from build123d import *

# Parameters (mm, degrees)
F0_W     = 25
F0_H     = 25
F1_DEPTH = 25
F3_R     = 5
F4_R     = 5


with BuildPart() as f1:
    # F0 (on Top) → F1 (new body)
    with BuildSketch(Plane.XY):
        with Locations((89.836757, -287.5)):
            Rectangle(F0_W, F0_H)
        with Locations((89.836757, -237.5)):
            Rectangle(F0_W, F0_H)
        with Locations((89.836757, -187.5)):
            Rectangle(F0_W, F0_H)
        with Locations((89.836757, -137.5)):
            Rectangle(F0_W, F0_H)
        with Locations((89.836757, -87.5)):
            Rectangle(F0_W, F0_H)
        with Locations((89.836757, -37.5)):
            Rectangle(F0_W, F0_H)
        Polygon((77.336757, 0), (-297.663243, 0), (-297.663243, -25), (-285.163243, -25), (-285.163243, -60), (-297.663243, -60), (-297.663243, -265), (-285.163243, -265), (-285.163243, -300), (-297.663243, -300), (-297.663243, -325), (77.336757, -325), (77.336757, -300), (77.336757, -275), (77.336757, -250), (77.336757, -225), (77.336757, -200), (77.336757, -175), (77.336757, -150), (77.336757, -125), (77.336757, -100), (77.336757, -75), (77.336757, -50), (77.336757, -25), align=None)
    extrude(amount=F1_DEPTH)

    # F2: F1 across face


with BuildPart() as f1_1:
    add(f1.part)
    add(f1.part.mirror(Plane(origin=(-297.663243, -162.5, 12.5), x_dir=(0, -1, 0), z_dir=(-1, 0, 0))))

    # F3
    f3_edges = [f1_1.edges().sort_by_distance(p)[0] for p in [
        (-297.663243, 0, 25),
    ]]
    fillet(f3_edges, radius=F3_R)

    # F4
    f4_edges = [f1_1.edges().sort_by_distance(p)[0] for p in [
        (-297.663243, -325, 25),
    ]]
    fillet(f4_edges, radius=F4_R)


solid = f1_1.part
Source: CAD feature listing. Evaluate the final solid. Frame: model axes, mm. A direction names the side the tool comes from. Round coordinates to 2 decimals unless told otherwise and drop trailing zeros. Write each loop counter-clockwise with the first axis right and the second up, starting at its lowest first coordinate (ties: lowest second). Pieces come first, ordered by that corner, then holes. Notation, with made-up numbers: M 61,43 L 67,43 A11 ccw 67,50 Z; hole C -11,-9.75 d3. An arc over 180 degrees is marked long. One line per item, written item: value. Start each with the question number.
Item 1: Section query A-A (z = 4.5). State how many separate pieces and enclosed holes the cut face has, plus the area to 4 significant figures.
Item 2: Set-up query: faces 1 (the flat face through (90, -225, 12)), 2 (the flat face through (-672.663, -113, 12)), 3 (the flat face through (-297, -25, 12)), 4 (the flat face through (77.337, -13, 12)). Return all of +Z, -Z, +X, -X, +Y, -Y with unobstructed straight access to the full face (end or side cutting, diameter ignored); none if empty.
Item 3: Section query B-B (y = -159.5). Return the cut outline in (x, z).
Item 4: Pin query (flat end, axial travel): pin 1 (5 mm diameter, centred on y = -153, z = 12, fed in from -X); pin 2 (6 mm diameter, centred on y = -107.5, z = 15.5, fed in from +X); pin 3 (7.5 mm diameter, centred on x = -687.5, z = 17, fed in from +Y). Return the tip coordinate at first contact, or that it passes through.
Item 5: Mould query, pull axis Y, two halves, no side actions, for faces 5 (the flat face through (90, -300, 12)), 6 (the flat face through (90, -50, 12)), 7 (the flat face through (102.337, -88, 12)). Classes: pulls with the +Y half, pulls with the -Y half, needs draft (parallel to the pull), parting line crosses it, or undercut.
Item 6: Ray query, L1, parallel to X at y = -29, z = 5.5; L2, parallel to X at y = -56, z = 11.75; L3, parallel to X at y = -253, z = 9.25. Return the intervals inside material, ascending. Write a range as from..to.
Result set:
1. separate pieces: 1
1. enclosed holes: 2
1. area: 249,500 mm²
2. face 1: +Z, -Z, +X
2. face 2: +Z, -Z, -X
2. face 3: +Z, -Z
2. face 4: +Z, -Z, +X, +Y
3. outline: M -672.66,0 L 77.34,0 L 77.34,25 L -672.66,25 Z
4. pin 1: stops at x = -672.66
4. pin 2: stops at x = 77.34
4. pin 3: stops at y = -25
5. face 5: pulls with the -Y half
5. face 6: undercut
5. face 7: needs draft
6. L1: x = -697.66..-310.16, -285.16..102.34
6. L2: x = -672.66..-310.16, -285.16..77.34
6. L3: x = -672.66..77.34
